from build123d import *

# Parameters (mm, degrees)
F0_W           = 50
F0_H           = 20
F1_DEPTH       = 25
F2_DEPTH       = 10
F4_DEPTH       = 50.001
F6_D           = 4.4
F6_CSINK_D     = 8.96
F6_CSINK_ANGLE = 90
F7_SIZE        = 0.5


with BuildPart() as f1:
    # F0 (on Top) → F1 (new body)
    with BuildSketch(Plane.XY):
        with Locations((0, 10)):
            Rectangle(F0_W, F0_H)
        with Locations((0, -10)):
            Rectangle(F0_W, F0_H)
    extrude(amount=F1_DEPTH)

    # F0 (on Top) → F2 (cut)
    with BuildSketch(Plane.XY):
        with Locations((0, 10)):
            Rectangle(F0_W, F0_H)
    extrude(amount=F2_DEPTH, mode=Mode.SUBTRACT)

    # F3 (on face) → F4 (cut, through all)
    with BuildSketch(Plane(origin=(-25, 0, 0), x_dir=(0, -1, 0), z_dir=(-1, 0, 0))):
        with BuildLine():
            ThreePointArc((10, 25), (17.0710678119, 22.0710678119), (20, 15))
            Line((20, 15), (20, 25))
            Line((20, 25), (10, 25))
        make_face()
    extrude(amount=-F4_DEPTH, mode=Mode.SUBTRACT)

    # F6 (through all)
    with Locations(Plane.XY.offset(25)):
        with Locations((0, 10)):
            CounterSinkHole(F6_D / 2, F6_CSINK_D / 2, counter_sink_angle=F6_CSINK_ANGLE)

    # F7
    f7_edges = [f1.edges().sort_by_distance(p)[0] for p in [
        (25, 20, 17.5),
        (-25, 20, 17.5),
    ]]
    chamfer(f7_edges, length=F7_SIZE)


solid = f1.part
Verification items for the finished model (mm, model axes). A direction names the side the tool comes from. Coordinates: 2 decimals unless noted, no trailing zeros. Order: outer loops, then holes, each group sorted by start corner. A loop starts at its lowest first (then second) coordinate and runs counter-clockwise, first axis right, second up. Notation, with made-up numbers: M 76,0.25 L 110,0.25 A21 cw 110,12.25 Z; hole C 48,57 d8. An arc over 180 degrees is marked long. Write each question's results on one line, items separated by ' | '.
1) Gauge pin test, flat ends, axial feed: pin 1 Ø5 at (x, y) = (-11.5, 12) entering from -Z; pin 2 Ø4 at (x, y) = (-11.5, -15.5) entering from +Z; pin 3 Ø7 at (x, y) = (0, 10) entering from +Z. Record the tip position at first contact, or that the pin passes through.
Solved:
pin 1: stops at z = 10 | pin 2: stops at z = 24.37 | pin 3: stops at z = 24.02
2) Section check B-B on x = 8. Record the cut outline in (y, z).
Solved:
outline: M -20,0 L 0,0 L 0,10 L 20,10 L 20,25 L -10,25 A10 ccw -20,15 Z
3) Section check C-C on x = 0. Record the cut outline in (y, z), plus the area to 3 significant figures.
Solved:
outline: M -20,0 L 0,0 L 0,10 L 7.8,10 L 7.8,22.72 L 5.52,25 L -10,25 A10 ccw -20,15 Z; M 12.2,10 L 20,10 L 20,25 L 14.48,25 L 12.2,22.72 Z | area: 707 mm²
4) Release check for a two-part mould opening along Y. For faces 1 (the face through (-0.3, 12.4, 10)), 2 (the face through (0, -20, 7)), 3 (the face through (-1.183, 11.855, 16.271)), 4 (the face through (0, 20, 17)) record: pulls with the +Y half, pulls with the -Y half, needs draft (parallel to the pull), parting line crosses it, or undercut.
Solved:
face 1: needs draft | face 2: pulls with the -Y half | face 3: undercut | face 4: pulls with the +Y half
5) Access from +Z, -Z, +X, -X, +Y, -Y to the whole of each face (thin tool, end or side, straight path). Record for faces 5 (the face through (0, 0, 5)), 6 (the face through (0.3, 12.29, 22.83)).
Solved:
face 5: -Z, +X, -X, +Y | face 6: +Z
6) Section check D-D on z = 3.25. Record the cut outline in (x, y).
Solved:
outline: M -25,-20 L 25,-20 L 25,0 L -25,0 Z
7) Scan lines: line 1 along X through (y, z) = (10, 17.5); line 2 along Y through (x, z) = (0, 13.25); line 3 along Y through (x, z) = (6, 1.75). Record each from-to range of solid material in increasing order. Write a range as [from, to].
Solved:
line 1: x = [-25, -2.2], [2.2, 25] | line 2: y = [-20, 7.8], [12.2, 20] | line 3: y = [-20, 0]
8) Section check A-A on y = 10. Record the cut outline in (x, z).
Solved:
outline: M -25,10 L -2.2,10 L -2.2,22.72 L -4.48,25 L -25,25 Z; M 2.2,10 L 25,10 L 25,25 L 4.48,25 L 2.2,22.72 Z
